```python
from build123d import *

# Parameters (mm, degrees)
F0_W     = 269.564176
F0_H     = 140
F1_DEPTH = 850
F3_DEPTH = 405.001
F4_R     = 118.296465
F5_R     = 147.774344
F6_DEPTH = 25


with BuildPart() as f1:
    # F0 (on Top) → F1 (new body)
    with BuildSketch(Plane.XY):
        Polygon((202.5, -230), (202.5, 230), (134.782088, 230), (-134.782088, 230), (-202.5, 230), (-202.5, -230), align=None)
        with Locations((0, 300)):
            Rectangle(F0_W, F0_H)
    extrude(amount=F1_DEPTH)

    # F2 (on face) → F3 (cut, through all)
    with BuildSketch(Plane.YZ.offset(202.5)):
        Polygon((-312.20004, 629.447699), (364.741862, 889.204443), (-312.20004, 956.11155), align=None)
    extrude(amount=-F3_DEPTH, mode=Mode.SUBTRACT)

    # F4
    f4_edges = [f1.edges().sort_by_distance(p)[0] for p in [
        (134.782088, 316.286348, 850),
        (-134.782088, 316.286348, 850),
    ]]
    fillet(f4_edges, radius=F4_R)

    # F5 (on face) → F6 (join)
    with BuildSketch(Plane(origin=(0, -250.602024, 653.084144), x_dir=(1, 0, 0), z_dir=(0, -0.358251, 0.933625))):
        with Locations((0, 327.743053)):
            Circle(F5_R)
    extrude(amount=F6_DEPTH)


solid = f1.part
```
The model under review builds one solid part; all positions refer to its coordinate system, in mm. A direction names the side the tool comes from. Coordinates: 2 decimals unless noted, no trailing zeros. Write each loop counter-clockwise with the first axis right and the second up, starting at its lowest first coordinate (ties: lowest second). Pieces come first, ordered by that corner, then holes.
1) We need section C-C on y = -152. State the section outline as (x, z) points, then the cut area to 3 significant figures.
2) We need section B-B on x = -104. State the section outline as (y, z) points, then the cut area to 3 significant figures.
3) We need section D-D on x = 47. State the section outline as (y, z) points, then the cut area to 3 significant figures.
4) Clearance check with flat-ended pins moving along their axes: pin 1 Ø2 at (x, y) = (-36.5, 292.5) entering from +Z; pin 2 Ø2 at (x, y) = (-102, 212.5) entering from +Z. State where each tip first meets the part, or that it passes through.
5) Machinability: for faces 1 (the face through (-101.049, 300.98, 814.427)), 2 (the face through (134.782, 299, 361)), 3 (the face through (-2.07, 48.36, 794.58)), 4 (the face through (101.049, 300.98, 814.427)), 5 (the face through (-134.782, 299, 361)), which of the approach directions +Z, -Z, +X, -X, +Y, -Y give a long, thin tool a straight path to every point of the face, cutting with its end or side? Answer none if there is none.
6) The part is to be moulded in two halves that separate along Y. For faces 6 (the face through (-3, 74, 0)), 7 (the face through (-3, -230, 326)), 8 (the face through (-32.035, -83.713, 730.324)), say which applies: pulls with the +Y half, pulls with the -Y half, needs draft (parallel to the pull), parting line crosses it, or undercut.
7) To check wall thickness, follow probe 1 along Y at (x, z) = (-171, 216.5); probe 2 along X at (y, z) = (270, 704.5); probe 3 along Z at (x, y) = (149.5, -110). State the ranges of each line that lie inside material, in increasing order.
8) We need section A-A on z = 551.5. State the section outline as (x, y) points.
Answer list:
1. outline: (-202.5, 0) - (202.5, 0) - (202.5, 690.92) - (-202.5, 690.92) - close
1. area: 280,000 mm2
2. outline: (-230, 0) - (370, 0) - (370, 811.3) - (230, 811.3) - (230, 837.5) - (153.4, 808.11) - (144.44, 831.45) - (-51.58, 756.23) - (-42.63, 732.89) - (-230, 660.99) - close
2. area: 463,000 mm2
3. outline: (-230, 0) - (370, 0) - (370, 846) - (252.14, 846) - (186.19, 820.69) - (177.23, 844.03) - (-84.37, 743.65) - (-75.41, 720.31) - (-230, 660.99) - close
3. area: 470,000 mm2
4. pin 1: stops at z = 848.46
4. pin 2: stops at z = 831.17
5. face 1: +Z, -X, +Y
5. face 2: +Z, -Z, +X, +Y
5. face 3: +Z, +X, -X, -Y
5. face 4: +Z, +X, +Y
5. face 5: +Z, -Z, -X, +Y
6. face 6: needs draft
6. face 7: pulls with the -Y half
6. face 8: undercut
7. probe 1: y = -230 to 230
7. probe 2: x = -134.78 to 134.78
7. probe 3: z = 0 to 707.04
8. outline: (-202.5, -230) - (202.5, -230) - (202.5, 230) - (134.78, 230) - (134.78, 370) - (-134.78, 370) - (-134.78, 230) - (-202.5, 230) - close
